Build history of the part. All positions in model axes, mm. Face numbers are marked on the shaded views. Coordinates: 2 decimals unless noted, no trailing zeros. Loops run counter-clockwise (first coordinate to the right, second up) from the corner with the lowest first, then second, coordinate; pieces in that order, holes last. Notation, with made-up numbers: (32.5, -22) - (37.5, -22) arc R30 ccw to (37.5, 8) - close; hole circle Ø9 at (-37.75, 88). An arc over 180 degrees is marked (long way). One line per item, written item: value.
```python
from build123d import *


with BuildPart() as f1:
    # F0 (on Front) → F1 (revolve)
    with BuildSketch(Plane.XZ):
        Polygon((0, 203.711763), (0, 0), (32.655226, 0), (32.655226, 33.276252), (14.980431, 33.276252), (14.980431, 45.901109), (32.655226, 45.901109), (32.655226, 57.263475), (14.980431, 57.263475), (14.980431, 67.363359), (32.655226, 67.363359), (32.655226, 140.587494), (14.980431, 140.587494), (14.980431, 153.212354), (32.655226, 153.212354), (32.655226, 165.837198), (14.980431, 165.837198), (14.980431, 177.199572), (32.655226, 177.199572), (32.655226, 188.561946), (14.980431, 188.561946), (50.33002, 203.711763), align=None)
        Polygon((32.655226, 0), (0, 0), (0, -203.711763), (50.33002, -203.711763), (14.980431, -188.561946), (32.655226, -188.561946), (32.655226, -177.199572), (14.980431, -177.199572), (14.980431, -165.837198), (32.655226, -165.837198), (32.655226, -153.212354), (14.980431, -153.212354), (14.980431, -140.587494), (32.655226, -140.587494), (32.655226, -67.363359), (14.980431, -67.363359), (14.980431, -57.263475), (32.655226, -57.263475), (32.655226, -45.901109), (14.980431, -45.901109), (14.980431, -33.276252), (32.655226, -33.276252), align=None)
    revolve(axis=Axis((0, 0, -101.855882), (0, 0, -1)))


solid = f1.part
```
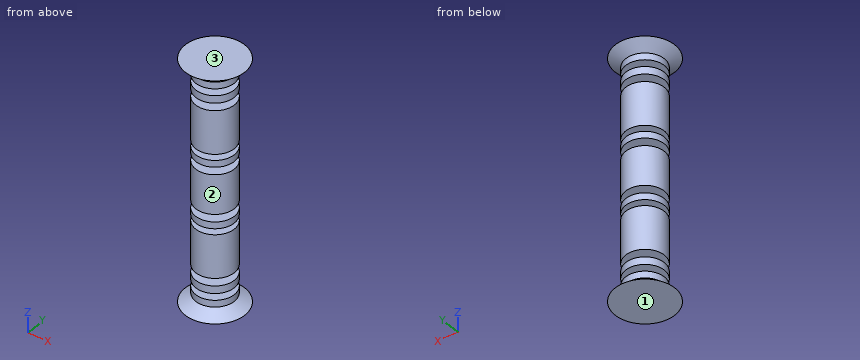
Item 1: Cut at B-B, the plane z = 41.5. Write the cut outline in (x, y), then the cut area to 3 significant figures.
Check result:
outline: circle Ø29.96 at (0, 0)
area: 705 mm^2
Item 2: Cut at A-A, the plane y = -24.5. Give the number of separate pieces and of enclosed holes in the cut face, then the cut area to 3 significant figures.
Check result:
separate pieces: 11
enclosed holes: 0
area: 13,500 mm^2
Item 3: Pull direction Z, two halves, no side cores. Call the marked faces 1, 2 and 3: released by +Z, released by -Z, zero draft, split by the parting line, or undercut.
Check result:
face 1: released by -Z
face 2: undercut
face 3: released by +Z
Item 4: Probe probe 1 along X at (y, z) = (2, 109); probe 2 along Z at (x, y) = (-37, 22); probe 3 along Z at (x, y) = (-46, -7). List the from-to ranges inside material, lowest first. Write a range as from..to.
Check result:
probe 1: x = -32.59..32.59
probe 2: z = -203.71..-200.59, 200.59..203.71
probe 3: z = -203.71..-202.08, 202.08..203.71
Item 5: Drop flat-ended pins along their axis: P1, Ø12, axis at y = -7, z = 34, coming from the +X side; P2, Ø8, axis at y = -8, z = -69.5, coming from the +X side; P3, Ø4, axis at x = 11, z = 149.5, coming from the -Y side. Give the stop position or say it passes through.
Check result:
P1: stops at x = 32.64
P2: stops at x = 32.41
P3: stops at y = -11.98
